For this review, take the finished solid that the model builds, in its own axes (mm). Face numbers are marked on the shaded views. A direction names the side the tool comes from. Give positions to 0.01 mm unless a question says otherwise; leave off trailing zeros. Write each loop counter-clockwise with the first axis right and the second up, starting at its lowest first coordinate (ties: lowest second). Pieces come first, ordered by that corner, then holes.
Q1. We need section B-B (y = 2.5). Write out the cut boundary in (x, z), then the cut area to 3 significant figures.
Q2. We need section A-A (z = 21). Write out the cut boundary in (x, y).
Q3. We need section D-D (x = -10). Write out the cut boundary in (y, z).
Q4. We need section C-C (y = 12). Give the number of separate pieces and of enclosed holes in the cut face, then the cut area to 3 significant figures.
Q5. Machinability: for the marked faces 4, 5 and 6, which of the approach directions +Z, -Z, +X, -X, +Y, -Y give a long, thin tool a straight path to every point of the face, cutting with its end or side? Answer none if there is none.
Q6. Mouldability with a two-part tool opening along X and no side actions: class the marked faces 1, 2 and 3 as released by +X, released by -X, zero draft, split by the parting line, or undercut.
Q7. For line 1 (Z direction, x = -10, y = 2.5); line 2 (Z direction, x = -10, y = -8); line 3 (Z direction, x = -10, y = 7.5), list the stretches that pass through material, from the lowest coordinate up.
Q8. Insertion check: P1, Ø3.5, axis at x = 9.5, y = 9.5, coming from the +Z side; P2, Ø3, axis at x = -2, z = 3, coming from the +Y side; P3, Ø4, axis at x = 15.5, z = 5.5, coming from the +Y side; P4, Ø8, axis at x = 4.5, z = -0.5, coming from the -Y side. Each pin has a flat end and moves straight along its axis. Give the tip position at first contact, or say it passes through.
Autodesk Inventor part; units mm, degrees
ref_plane "Work Plane2" through (11, 18, -30) normal (1, 0, 0) x (0, 1, 0)
ref_plane "XZ Plane" through (0, 0, 0) normal (0, 1, 0) x (-1, 0, 0)
ref_plane "XY Plane" through (0, 0, 0) normal (0, 0, 1) x (1, 0, 0)
sketch "Sketch1" plane through (0, 0, 0) normal (0, 1, 0) x (-1, 0, 0)
  line L0 (-25, 30) -> (25, 30)
  line L1 (25, 30) -> (25, -30)
  line L2 (25, -30) -> (-25, -30)
  line L3 (-25, -30) -> (-25, 30)
  line L4 (-25, 30) -> (25, -30) construction
  line L5 (25, 30) -> (-25, -30) construction
  point P0 (0, 0)
  dimension "d0" = 50
  dimension "d1" = 60
extrude "Extrusion1" add sketch "Sketch1" along normal blind 18
sketch "Sketch2" plane through (25, 0, 30) normal (1, 0, 0) x (0, 0, -1)
  line L0 (60, 18) -> (0, 18)
  circle A0 centre (30, 18) radius 9.5
  point P0 (30, 0)
  point P1 (20.5, 18)
  point P2 (39.5, 18)
  dimension "d4" = 19
extrude "Extrusion2" cut sketch "Sketch2" against normal through all contours A0 L0 picked at (28.8771, 15.0391)
sketch "Sketch3" plane through (25, 0, -30) normal (0, 0, -1) x (-1, 0, 0)
  line L0 (0, 18) -> (50, 18)
  circle A0 centre (14, 18) radius 10
  point P0 (25, 0)
  point P1 (24, 18)
  point P2 (4, 18)
  dimension "d7" = 20
  dimension "d8" = 14
extrude "Extrusion3" cut sketch "Sketch3" against normal through all contours L0 A0 picked at (12.1065, 15.2567)
sketch "Sketch4" plane through (0, 0, 0) normal (0, 0, 1) x (1, 0, 0)
  arc A0 (1, 18) -> (21, 18) centre (11, 18) ccw
  circle A1 centre (11, 18) radius 11.5
  point P0 (0, 0)
  dimension "d11" = 23
extrude "Extrusion4" cut sketch "Sketch4" along normal mid plane 39
ref_plane "Work Plane2" through (11, 18, -30) normal (1, 0, 0) x (0, 1, 0)
sketch "Sketch5" plane through (11, 18, -30) normal (1, 0, 0) x (0, 1, 0)
  arc A0 (0, 39.5) -> (0, 20.5) centre (0, 30) ccw
  circle A1 centre (0, 30) radius 11.5
  point P0 (-18, 30)
  dimension "d14" = 23
extrude "Extrusion5" cut sketch "Sketch5" against normal blind 24
sketch "Sketch7" plane through (0, 0, 0) normal (0, -1, 0) x (1, 0, 0)
  line L0 (25, -30) -> (-25, -30)
  line L1 (-25, 30) -> (25, 30)
  line L2 (-25, -30) -> (-25, 30)
  point P0 (0, 0)
  point P1 (-10, -21)
  point P2 (-10, 21)
  dimension "d28" = 9
  dimension "d29" = 9
  dimension "d30" = 15
hole "Hole2" at (-10, 0, -21) at (-10, 0, 21) direction (0, 1, 0) diameter 6.756 end through all
fillet "Fillet1" radius 5 4 edges at (-25, 9, -30) (-25, 9, 30) (25, 9, 30) (25, 9, -30)
mirror "Mirror1" about plane through (0, 0, 0) normal (0, -1, 0)
properties part number "Valve Block Middle"
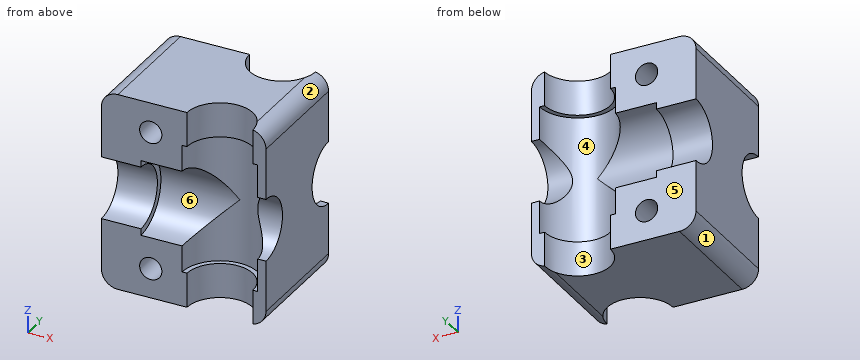
Computed:
1. outline: (-25, -25) arc R5 ccw to (-20, -30) - (20, -30) arc R5 ccw to (25, -25) - (25, 25) arc R5 ccw to (20, 30) - (-20, 30) arc R5 ccw to (-25, 25) - close; hole circle Ø6.76 at (-10, -21); hole circle Ø6.76 at (-10, 21)
1. area: 2,910 mm2
2. outline: (-25, -18) - (-13.38, -18) - (-13.38, 18) - (-25, 18) - close; (-6.62, -18) - (1, -18) arc R10 cw to (21, -18) - (25, -18) - (25, 18) - (21, 18) arc R10 cw to (1, 18) - (-6.62, 18) - close
3. outline: (-18, -30) - (18, -30) - (18, -24.38) - (-18, -24.38) - close; (-18, -17.62) - (18, -17.62) - (18, -11.5) arc R11.5 cw to (18, 11.5) - (18, 17.62) - (-18, 17.62) - (-18, 11.5) arc R11.5 cw to (-18, -11.5) - close; (-18, 24.38) - (18, 24.38) - (18, 30) - (-18, 30) - close
4. separate pieces: 4
4. enclosed holes: 2
4. area: 1,290 mm2
5. face 4: +Y
5. face 5: +Z, -Z, +X, -X, +Y
5. face 6: -Y
6. face 1: released by -X
6. face 2: released by +X
6. face 3: undercut
7. line 1: z = -30 to -24.38, -17.62 to 17.62, 24.38 to 30
7. line 2: z = -30 to -24.38, -17.62 to -5.68, 5.68 to 17.62, 24.38 to 30
7. line 3: z = -30 to -24.38, -17.62 to -4.69, 4.69 to 17.62, 24.38 to 30
8. P1: stops at z = 30
8. P2: stops at y = 7.42
8. P3: stops at y = 8.51
8. P4: stops at y = -7.42
